Check sheet for the modelled part. Datum: model origin and axes. Units: mm. A direction names the side the tool comes from. Give positions to 0.01 mm unless a question says otherwise; leave off trailing zeros. Write each loop counter-clockwise with the first axis right and the second up, starting at its lowest first coordinate (ties: lowest second). Pieces come first, ordered by that corner, then holes. Notation, with made-up numbers: (-3, 35.5) -> (13, 35.5) arc R32 cw to (13, 70.5) -> close; hole circle Ø4 at (7, 43). An arc over 180 degrees is marked (long way). Use a Markdown table: item, result. Add a question column.
1. Cross-section at C-C (z = -10). Enter the section's corners in (x, y).
2. Release check for a two-part mould opening along Z. For faces 1 (the cylindrical face through (-37.014, 37.747, -9.879)), 2 (the flat face through (-18, -1, 0)), 3 (the flat face through (35, -1, -10)), 4 (the cylindrical face through (26.419, -1.014, -8.452)) record: released by +Z, released by -Z, zero draft, split by the parting line, or undercut.
3. Scan lines: probe 1 along Z at (x, y) = (-36.7, 10); probe 2 along X at (y, z) = (-0.8, -10); probe 3 along X at (y, z) = (-1.35, -10). Record each from-to range of solid material in increasing order. Write a range as [from, to].
4. Set-up check for faces 5 (the cylindrical face through (-37.1, -1.14, -10.14)), 6 (the flat face through (-0.5, 0, -12.4)): record each of +Z, -Z, +X, -X, +Y, -Y from which the full face is reachable in a straight line by a thin tool's end or side.
5. Gauge pin test, flat ends, axial feed: P1, Ø8, axis at x = -0.5, z = -11.5, coming from the +Y side; P2, Ø7, axis at y = 35, z = -10, coming from the +X side; P3, Ø4.5, axis at y = 10, z = -10, coming from the -X side. Record the tip position at first contact, or that the pin passes through.
6. Cross-section at D-D (z = -1.75). Enter the section's corners in (x, y), then the cut area to 3 significant figures.
7. Cross-section at B-B (y = 10). Enter the section's corners in (x, z).
8. Cross-section at A-A (x = 0). Enter the section's corners in (y, z), then the cut area to 3 significant figures.
from build123d import *

# Parameters (mm, degrees)
SKETCH_1_W             = 70
SKETCH_1_H             = 20
SM_BASE_FLANGE_1_DEPTH = 2
SM_EDGE_FLANGE_1_DEPTH = 20
MM_1_D                 = 5.5
MM_1_DEPTH             = 8
MM_1_TIP               = 1.652366702
HOLE_WIZARD_M5_1_D     = 4.2
HOLE_WIZARD_M5_1_DEPTH = 12.4
HOLE_WIZARD_M5_1_TIP   = 1.2618073


# Sheet-metal steps are written as plain solids
with BuildPart() as part:
    # Sketch 1 → 基体-法兰1 (new body)
    with BuildSketch(Plane(origin=(0, 0, 0), x_dir=(1, 0, 0), z_dir=(0, 1, 0))):
        with Locations((0, 10)):
            Rectangle(SKETCH_1_W, SKETCH_1_H)
    extrude(amount=-SM_BASE_FLANGE_1_DEPTH)

    # 边线-法兰1 section (across the edge) → 边线-法兰1 (add)
    with BuildSketch(Plane(origin=(-36, 0, -20), x_dir=(1, 0, 0), z_dir=(0, 0, 1))):
        with BuildLine():
            Line((-2, 1), (-2, 43))
            Line((-2, 43), (0, 43))
            Line((0, 43), (0, 1))
            ThreePointArc((0, 1), (0.292893219, 0.292893219), (1, 0))
            Line((1, 0), (1, -2))
            ThreePointArc((1, -2), (-1.121320344, -1.121320344), (-2, 1))
        make_face()
    extrude(amount=SM_EDGE_FLANGE_1_DEPTH)

    # 大小mm 暗销孔1
    with Locations(Plane(origin=(-36, 35, -10), x_dir=(0, 1, 0), z_dir=(1, 0, 0))):
        with Locations((0, 0), (-25, 0)):
            Hole(MM_1_D / 2, depth=MM_1_DEPTH)
            with Locations((0, 0, -(MM_1_DEPTH + MM_1_TIP / 2))):  # 118° drill point
                Cone(0, MM_1_D / 2, MM_1_TIP, mode=Mode.SUBTRACT)

    # M5 螺纹孔1
    with Locations(Plane(origin=(0, 0, -10), x_dir=(0, 0, 1), z_dir=(0, 1, 0))):
        with Locations((0, 0), (0, 25), (-27.106002663, 33.534976499)):
            Hole(HOLE_WIZARD_M5_1_D / 2, depth=HOLE_WIZARD_M5_1_DEPTH)
            with Locations((0, 0, -(HOLE_WIZARD_M5_1_DEPTH + HOLE_WIZARD_M5_1_TIP / 2))):  # 118° drill point
                Cone(0, HOLE_WIZARD_M5_1_D / 2, HOLE_WIZARD_M5_1_TIP, mode=Mode.SUBTRACT)


solid = part.part
Worked answers:
| question | item | result |
|---|---|---|
| 1 | outline | (-38, 1) arc R3 ccw to (-35, -2) -> (-2.1, -2) -> (-2.1, 0) -> (-35, 0) arc R1 cw to (-36, 1) -> (-36, 7.25) -> (-38, 7.25) -> close; (-38, 12.75) -> (-36, 12.75) -> (-36, 32.25) -> (-38, 32.25) -> close; (-38, 37.75) -> (-36, 37.75) -> (-36, 43) -> (-38, 43) -> close; (2.1, -2) -> (22.9, -2) -> (22.9, 0) -> (2.1, 0) -> close; (27.1, -2) -> (35, -2) -> (35, 0) -> (27.1, 0) -> close |
| 2 | face 1 | undercut |
| 2 | face 2 | released by +Z |
| 2 | face 3 | zero draft |
| 2 | face 4 | undercut |
| 3 | probe 1 | z = [-20, -12.75], [-7.25, 0] |
| 3 | probe 2 | x = [-37.4, -2.1], [2.1, 22.9], [27.1, 35] |
| 3 | probe 3 | x = [-36.86, -2.1], [2.1, 22.9], [27.1, 35] |
| 4 | face 5 | +Z, -Z, -X, -Y |
| 4 | face 6 | +Z, -Z, +X, +Y |
| 5 | P1 | stops at y = 0 |
| 5 | P2 | stops at x = -36 |
| 5 | P3 | passes through |
| 6 | outline | (-38, 1) arc R3 ccw to (-35, -2) -> (35, -2) -> (35, 0) -> (-35, 0) arc R1 cw to (-36, 1) -> (-36, 43) -> (-38, 43) -> close |
| 6 | area | 230 mm² |
| 7 | outline | (-38, -20) -> (-36, -20) -> (-36, -12.75) -> (-38, -12.75) -> close; (-38, -7.25) -> (-36, -7.25) -> (-36, 0) -> (-38, 0) -> close |
| 8 | outline | (-2, -20) -> (0, -20) -> (0, -12.1) -> (-2, -12.1) -> close; (-2, -7.9) -> (0, -7.9) -> (0, 0) -> (-2, 0) -> close |
| 8 | area | 31.6 mm² |
